The listing builds one solid part. Answer for the finished solid, in the listing's coordinates (mm). A direction names the side the tool comes from. Coordinates: 2 decimals unless noted, no trailing zeros. Order: outer loops, then holes, each group sorted by start corner. A loop starts at its lowest first (then second) coordinate and runs counter-clockwise, first axis right, second up. Notation, with made-up numbers: (-35, -1) -> (0, -1) arc R24 cw to (0, 19) -> close; hole circle Ø9 at (-9, 57). An arc over 180 degrees is marked (long way). Answer in a Markdown table with one row per item.
Autodesk Inventor part; units mm, degrees
ref_plane "YZ Plane" through (0, 0, 0) normal (1, 0, 0) x (0, 1, 0)
ref_plane "XZ Plane" through (0, 0, 0) normal (0, 1, 0) x (-1, 0, 0)
ref_plane "XY Plane" through (0, 0, 0) normal (0, 0, 1) x (1, 0, 0)
sketch "Sketch1" plane through (0, 0, 0) normal (0, 0, 1) x (1, 0, 0)
  circle A0 centre (0, 0) radius 4.59
  arc A1 (-2.0962, 20.2222) -> (2.0962, 39.7778) centre (0, 30) ccw
  line L0 (2.0962, 39.7778) -> (-22.6062, 45.0736)
  line L1 (-2.0962, 20.2222) -> (-43.8842, 29.1807)
  line L2 (50, -20) -> (50, 20)
  arc A2 (-46.0074, 28.2723) -> (49.8462, -20.7692) centre (0, 0) ccw
  arc A3 (49.8462, 20.7692) -> (-23.0403, 48.8379) centre (0, 0) ccw
  arc A4 (-43.8842, 29.1807) -> (-46.0074, 28.2723) centre (-44.3034, 27.2252) ccw
  arc A5 (-23.0403, 48.8379) -> (-22.6062, 45.0736) centre (-22.187, 47.0291) ccw
  arc A6 (50, 20) -> (49.8462, 20.7692) centre (48, 20) ccw
  arc A7 (49.8462, -20.7692) -> (50, -20) centre (48, -20) ccw
  point P0 (-27.9313, 46.2152)
  point P1 (-45.2476, 29.473)
  point P2 (50, -20.3961)
  point P3 (50, 20.3961)
  dimension "d1" = 9.18
  dimension "d4" = 20
  dimension "d5" = 30
  dimension "d12" = 50
  dimension "d13" = 2
  dimension "d14" = 54
  dimension "d15" = 54
  dimension "d16" = 20
  dimension "d19" = 77.9
  dimension "d20" = 50
extrude "Extrusion3" add sketch "Sketch1" along normal blind 3
properties part number "OpenROV 2_3_2 Dev EndCap 108"
(1) A cutting plane is placed at B-B, the plane z = 1.5. Determine the outline of the cut face in (x, y), then the cut area to 3 significant figures.
Check values:
| item | result |
|---|---|
| outline | (-46.01, 28.27) arc R54 ccw (long way) to (49.85, -20.77) arc R2 ccw to (50, -20) -> (50, 20) arc R2 ccw to (49.85, 20.77) arc R54 ccw to (-23.04, 48.84) arc R2 ccw to (-22.61, 45.07) -> (2.1, 39.78) arc R10 cw to (-2.1, 20.22) -> (-43.88, 29.18) arc R2 ccw to start; hole circle Ø9.18 at (0, 0) |
| area | 8,050 mm² |
(2) A cutting plane is placed at D-D, the plane y = -47. Determine the outline of the cut face in (x, z), then the cut area to 3 significant figures.
Check values:
| item | result |
|---|---|
| outline | (-26.59, 0) -> (26.59, 0) -> (26.59, 3) -> (-26.59, 3) -> close |
| area | 160 mm² |
(3) A cutting plane is placed at A-A, the plane y = 0. Determine the outline of the cut face in (x, z).
Check values:
| item | result |
|---|---|
| outline | (-54, 0) -> (-4.59, 0) -> (-4.59, 3) -> (-54, 3) -> close; (4.59, 0) -> (50, 0) -> (50, 3) -> (4.59, 3) -> close |
(4) Find the intervals of material crossed by line 1 along X through (y, z) = (0.5, 1.95); line 2 along Y through (x, z) = (0, 0.9); line 3 along Y through (x, z) = (8.5, 0.6), in increasing order. Write a range as from..to.
Check values:
| item | result |
|---|---|
| line 1 | -54..-4.56, 4.56..50 |
| line 2 | -54..-4.59, 4.59..20, 40.23..54 |
| line 3 | -53.33..24.73, 35.27..53.33 |
(5) A cutting plane is placed at C-C, the plane x = 0. Determine the outline of the cut face in (y, z), then the cut area to 3 significant figures.
Check values:
| item | result |
|---|---|
| outline | (-54, 0) -> (-4.59, 0) -> (-4.59, 3) -> (-54, 3) -> close; (4.59, 0) -> (20, 0) -> (20, 3) -> (4.59, 3) -> close; (40.23, 0) -> (54, 0) -> (54, 3) -> (40.23, 3) -> close |
| area | 236 mm² |
(6) Which of the six approach directions +Z, -Z, +X, -X, +Y, -Y give full straight-line access (tool end or side, diameter ignored) to faces 4 (the flat face through (-10.08, 42.39, 1.48)), 5 (the cylindrical face through (-1, 4.48, 1.48))?
Check values:
| item | result |
|---|---|
| face 4 | +Z, -Z, -X |
| face 5 | +Z, -Z |
(7) Flat-ended cylindrical pins translate along their axes: pin 1 (12 mm diameter, centred on x = 0, y = 0, fed in from +Z); pin 2 (1 mm diameter, centred on y = 34.5, z = 2, fed in from -X); pin 3 (1 mm diameter, centred on x = -13.5, z = 2.5, fed in from -Y); pin 4 (1.5 mm diameter, centred on y = 38.5, z = 2, fed in from -X). Find the tip coordinate at first contact, or state that the pin passes through.
Check values:
| item | result |
|---|---|
| pin 1 | z = 3 |
| pin 2 | x = 8.66 |
| pin 3 | y = -52.41 |
| pin 4 | x = 3.8 |
(8) For a pull along Y with two mould halves and no side action, classify faces 1 (the cylindrical face through (-23.48, -48.63, 1.48)), 2 (the flat face through (-22.7, 24.64, 1.48)), 3 (the flat face through (-3, -11, 3)) as released by +Y, released by -Y, zero draft, split by the parting line, or undercut.
Check values:
| item | result |
|---|---|
| face 1 | split by the parting line |
| face 2 | undercut |
| face 3 | zero draft |
